Geometry: final body of the model. Coordinates: model frame, mm. Give positions to 0.01 mm unless a question says otherwise; leave off trailing zeros. Write each loop counter-clockwise with the first axis right and the second up, starting at its lowest first coordinate (ties: lowest second). Pieces come first, ordered by that corner, then holes. Notation, with made-up numbers: M 1.5,64.25 L 60.5,64.25 A15 ccw 60.5,92.25 Z; hole C 26,-6.5 d8. An arc over 180 degrees is marked long. One line per question, with ' | ' between items.
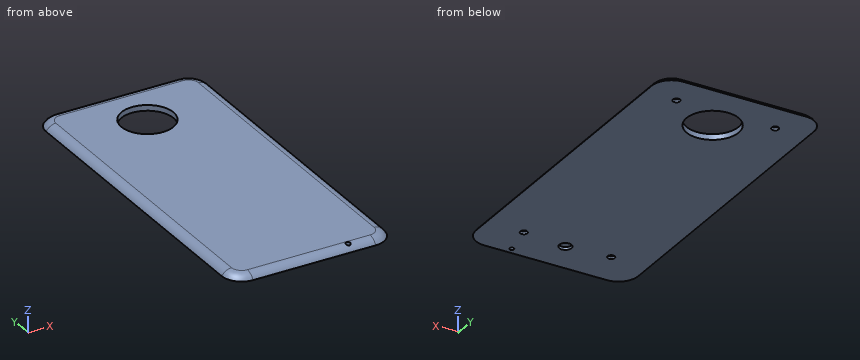
from build123d import *

# Parameters (mm, degrees)
F1_DEPTH     = 2.54
F2_R         = 11.75
F3_DEPTH     = 2.541
F4_R         = 8.89
F5_T1_DEPTH  = 135.128
F5_T3_DEPTH  = 55.372
F5_T6_ANGLE  = 90
F5_T8_ANGLE  = 90
F5_T10_ANGLE = 90
F5_T12_ANGLE = 90
F6_R         = 1
F7_DEPTH     = 2.541
F9_R         = 1.6
F8_R         = 1.6
F10_DEPTH    = 1.2
F11_R        = 2.794
F12_DEPTH    = 1.27


# Not quite as in the source:
# - a fillet or chamfer that OpenCascade refuses, or shapes differently, is made with other operations: its cross-section is extruded or revolved along the edge and cut away or added


with BuildPart() as f1:
    # F0 (on Top) → F1 (new body)
    with BuildSketch(Plane.XY):
        Polygon((36.576, 76.454), (0, 76.454), (-36.576, 76.454), (-36.576, 0), (-36.576, -76.454), (0, -76.454), (36.576, -76.454), (36.576, 0), align=None)
    extrude(amount=F1_DEPTH)

    # F2 (on face) → F3 (cut, through all)
    with BuildSketch(Plane.XY.offset(2.54)):
        with Locations((0, 52.004)):
            Circle(F2_R)
    extrude(amount=-F3_DEPTH, mode=Mode.SUBTRACT)

    # F4
    f4_edges = [f1.edges().sort_by_distance(p)[0] for p in [
        (-36.576, 76.454, 1.27),
        (36.576, 76.454, 1.27),
        (36.576, -76.454, 1.27),
        (-36.576, -76.454, 1.27),
    ]]
    fillet(f4_edges, radius=F4_R)

    # F5: fillet of radius 5.08 on 1 edges, made by hand

    # F5_s2 → F5_t1 (cut)
    with BuildSketch(Plane.XZ.offset(-67.564)):
        with BuildLine():
            ThreePointArc((32.1765909488, 2.54), (34.7165909488, 1.8594090512), (36.576, 0))
            Line((36.576, 0), (36.576, 2.54))
            Line((36.576, 2.54), (32.1765909488, 2.54))
        make_face()
        with BuildLine():
            ThreePointArc((-32.1765909488, 2.54), (-34.7165909488, 1.8594090512), (-36.576, 0))
            Line((-36.576, 0), (-36.576, 2.54))
            Line((-36.576, 2.54), (-32.1765909488, 2.54))
        make_face()
    extrude(amount=F5_T1_DEPTH, mode=Mode.SUBTRACT)

    # F5_s4 → F5_t3 (cut)
    with BuildSketch(Plane.YZ.offset(-27.686)):
        with BuildLine():
            ThreePointArc((-72.0545909488, 2.54), (-74.5945909488, 1.8594090512), (-76.454, 0))
            Line((-76.454, 0), (-76.454, 2.54))
            Line((-76.454, 2.54), (-72.0545909488, 2.54))
        make_face()
        with BuildLine():
            ThreePointArc((76.454, 0), (74.5945909488, 1.8594090512), (72.0545909488, 2.54))
            Line((72.0545909488, 2.54), (76.454, 2.54))
            Line((76.454, 2.54), (76.454, 0))
        make_face()
    extrude(amount=F5_T3_DEPTH, mode=Mode.SUBTRACT)

    # F5_s5 → F5_t6 (revolve, cut)
    with BuildSketch(Plane.YZ.offset(27.686)):
        with BuildLine():
            ThreePointArc((72.0545909488, 2.54), (74.5945909488, 1.8594090512), (76.454, 0))
            Line((76.454, 0), (76.454, 2.54))
            Line((76.454, 2.54), (72.0545909488, 2.54))
        make_face()
    revolve(axis=Axis((27.686, 67.564, 2.54), (0, 0, -1)), revolution_arc=F5_T6_ANGLE, mode=Mode.SUBTRACT)

    # F5_s7 → F5_t8 (revolve, cut)
    with BuildSketch(Plane.XZ.offset(67.564)):
        with BuildLine():
            ThreePointArc((32.1765909488, 2.54), (34.7165909488, 1.8594090512), (36.576, 0))
            Line((36.576, 0), (36.576, 2.54))
            Line((36.576, 2.54), (32.1765909488, 2.54))
        make_face()
    revolve(axis=Axis((27.686, -67.564, 2.54), (0, 0, -1)), revolution_arc=F5_T8_ANGLE, mode=Mode.SUBTRACT)

    # F5_s9 → F5_t10 (revolve, cut)
    with BuildSketch(Plane.XZ.offset(67.564)):
        with BuildLine():
            ThreePointArc((-32.1765909488, 2.54), (-34.7165909488, 1.8594090512), (-36.576, 0))
            Line((-36.576, 0), (-36.576, 2.54))
            Line((-36.576, 2.54), (-32.1765909488, 2.54))
        make_face()
    revolve(axis=Axis((-27.686, -67.564, 2.54), (0, 0, 1)), revolution_arc=F5_T10_ANGLE, mode=Mode.SUBTRACT)

    # F5_s11 → F5_t12 (revolve, cut)
    with BuildSketch(Plane.YZ.offset(-27.686)):
        with BuildLine():
            ThreePointArc((72.0545909488, 2.54), (74.5945909488, 1.8594090512), (76.454, 0))
            Line((76.454, 0), (76.454, 2.54))
            Line((76.454, 2.54), (72.0545909488, 2.54))
        make_face()
    revolve(axis=Axis((-27.686, 67.564, 2.54), (0, 0, 1)), revolution_arc=F5_T12_ANGLE, mode=Mode.SUBTRACT)

    # F6 (on face) → F7 (cut, through all)
    with BuildSketch(Plane(origin=(0, 0, 0), x_dir=(1, 0, 0), z_dir=(0, 0, -1))):
        with Locations((17.018, 73.406)):
            Circle(F6_R)
    extrude(amount=-F7_DEPTH, mode=Mode.SUBTRACT)

    # F9 (on face) + F8 (on face) → F10 (cut)
    with BuildSketch(Plane(origin=(0, 0, 0), x_dir=(1, 0, 0), z_dir=(0, 0, -1))):
        with Locations((19.736, 59.614)):
            Circle(F9_R)
        with Locations((-19.736, 59.614)):
            Circle(F9_R)
    with BuildSketch(Plane(origin=(0, 0, 0), x_dir=(1, 0, 0), z_dir=(0, 0, -1))):
        with Locations((-22.276, -62.154)):
            Circle(F8_R)
        with Locations((22.276, -62.154)):
            Circle(F8_R)
    extrude(amount=-F10_DEPTH, mode=Mode.SUBTRACT)

    # F11 (on face) → F12 (cut)
    with BuildSketch(Plane(origin=(0, 0, 0), x_dir=(1, 0, 0), z_dir=(0, 0, -1))):
        with Locations((0, 61.214)):
            Circle(F11_R)
    extrude(amount=-F12_DEPTH, mode=Mode.SUBTRACT)


solid = f1.part
(1) First-contact query: P1, Ø4.5, axis at x = 0, y = -61.5, coming from the -Z side; P2, Ø1.8, axis at x = 17.018, y = -73.406, coming from the -Z side; P3, Ø2.5, axis at x = -22, y = 62, coming from the -Z side; P4, Ø1, axis at y = -27, z = 2, coming from the -X side. Flat tips, straight axial feed; report the tip coordinate or a pass-through.
Working result:
P1: stops at z = 1.27 | P2: passes through | P3: stops at z = 1.2 | P4: stops at x = -35.26
(2) Cut plane D-D, the plane y = 21. Return loops of the section in (x, z), then the cut area to 3 significant figures.
Working result:
outline: M -36.58,0 L 36.58,0 A5.08 ccw 32.18,2.54 L -32.18,2.54 A5.08 ccw Z | area: 179 mm^2
(3) Cut plane C-C, the plane x = 9. Return loops of the section in (y, z), then the cut area to 3 significant figures.
Working result:
outline: M -76.45,0 L 44.45,0 L 44.45,2.54 L -72.05,2.54 A5.08 ccw Z; M 59.56,0 L 76.45,0 A5.08 ccw 72.05,2.54 L 59.56,2.54 Z | area: 344 mm^2
(4) Material intervals for L1, parallel to Y at x = -21, z = 1.05; L2, parallel to Y at x = 3.5, z = 1.4; L3, parallel to Y at x = 9, z = 1.4, sorted ascending. Write a range as [from, to].
Working result:
L1: y = [-75.65, -60.59], [-58.63, 61.19], [63.12, 75.65] | L2: y = [-75.26, 40.79], [63.22, 75.26] | L3: y = [-75.26, 44.45], [59.56, 75.26]
(5) Cut plane B-B, the plane y = 59. Return loops of the section in (x, z).
Working result:
outline: M -36.58,0 L -9.44,0 L -9.44,2.54 L -32.18,2.54 A5.08 ccw Z; M 9.44,0 L 36.58,0 A5.08 ccw 32.18,2.54 L 9.44,2.54 Z
(6) Cut plane A-A, the plane x = 0. Return loops of the section in (y, z), then the cut area to 3 significant figures.
Working result:
outline: M -76.45,0 L -64.01,0 L -64.01,1.27 L -58.42,1.27 L -58.42,0 L 40.25,0 L 40.25,2.54 L -72.05,2.54 A5.08 ccw Z; M 63.75,0 L 76.45,0 A5.08 ccw 72.05,2.54 L 63.75,2.54 Z | area: 315 mm^2
